from build123d import *

# Parameters (mm, degrees)
SKETCH1_R             = 14.2875
BOSS_EXTRUDE1_DEPTH   = 3.175
F_5_0MM_DOWEL_HOLE1_D = 5


with BuildPart() as part:
    # Sketch1 → Boss-Extrude1 (new, symmetric)
    with BuildSketch(Plane.XY):
        with BuildLine():
            Line((-5.294178862, 26.506304348), (-15.882536585, 10.518913043))
            ThreePointArc((-15.882536585, 10.518913043), (-19.05, 0), (-15.882536585, -10.518913043))
            Line((-15.882536585, -10.518913043), (-5.294178862, -26.506304348))
            ThreePointArc((-5.294178862, -26.506304348), (0, -29.35), (5.294178862, -26.506304348))
            Line((5.294178862, -26.506304348), (15.882536585, -10.518913043))
            ThreePointArc((15.882536585, -10.518913043), (19.05, 0), (15.882536585, 10.518913043))
            Line((15.882536585, 10.518913043), (5.294178862, 26.506304348))
            ThreePointArc((5.294178862, 26.506304348), (0, 29.35), (-5.294178862, 26.506304348))
        make_face()
        Circle(SKETCH1_R, mode=Mode.SUBTRACT)
    extrude(amount=BOSS_EXTRUDE1_DEPTH, both=True)

    # Ø5.0mm Dowel Hole1 (through all)
    with Locations(Plane.XY.offset(3.175)):
        with Locations((0, 23), (0, -23)):
            Hole(F_5_0MM_DOWEL_HOLE1_D / 2)


solid = part.part
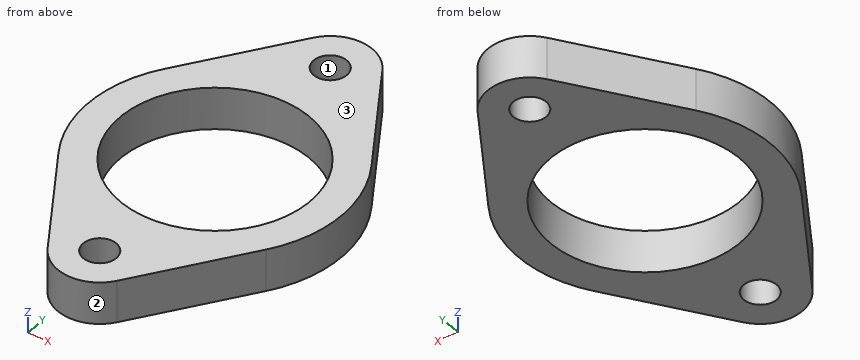
The model under review builds one solid part; all positions refer to its coordinate system, in mm. Face numbers are marked on the shaded views. Coordinates: 2 decimals unless noted, no trailing zeros. Loops run counter-clockwise (first coordinate to the right, second up) from the corner with the lowest first, then second, coordinate; pieces in that order, holes last. Notation, with made-up numbers: (5.25, 87) -> (10.25, 87) arc R31 cw to (10.25, 117) -> close; hole circle Ø8 at (44, -14). An arc over 180 degrees is marked (long way). Use a Markdown table: item, result. Add a question column.
1. To check wall thickness, follow line 1 (Y direction, x = -2, z = -1); line 2 (Y direction, x = 9.5, z = -0.5); line 3 (Y direction, x = 8, z = -0.25). State the ranges of each line that lie inside material, in increasing order.
2. Add section B-B on x = 0. Give the number of separate pieces and of enclosed holes in the cut face, plus the area to 3 significant figures.
3. Clearance check with flat-ended pins moving along their axes: pin 1 Ø4 at (x, y) = (0, -23) entering from -Z; pin 2 Ø3 at (y, z) = (-8, 2) entering from -X; pin 3 Ø2 at (y, z) = (6.5, 0) entering from +X. State where each tip first meets the part, or that it passes through.
4. Draft analysis for pull direction X (two halves, no side actions). For the marked faces 1, 2 and 3, state which applies: pulls with the +X half, pulls with the -X half, needs draft (parallel to the pull), parting line crosses it, or undercut.
5. Add section C-C on x = -11.5. Write out the cut boundary in (y, z) (3 decimals), plus the area to 3 significant figures.
Returned:
| question | item | result |
|---|---|---|
| 1 | line 1 | y = -29.03 to -24.5, -21.5 to -14.15, 14.15 to 21.5, 24.5 to 29.03 |
| 1 | line 2 | y = -20.16 to -10.67, 10.67 to 20.16 |
| 1 | line 3 | y = -22.42 to -11.84, 11.84 to 22.42 |
| 2 | separate pieces | 4 |
| 2 | enclosed holes | 0 |
| 2 | area | 128 mm² |
| 3 | pin 1 | passes through |
| 3 | pin 2 | stops at x = -17.91 |
| 3 | pin 3 | stops at x = 18.24 |
| 4 | face 1 | undercut |
| 4 | face 2 | parting line crosses it |
| 4 | face 3 | needs draft |
| 5 | outline | (-17.136, -3.175) -> (-8.478, -3.175) -> (-8.478, 3.175) -> (-17.136, 3.175) -> close; (8.478, -3.175) -> (17.136, -3.175) -> (17.136, 3.175) -> (8.478, 3.175) -> close |
| 5 | area | 110 mm² |
